For this review, take the finished solid that the model builds, in its own axes (mm). A direction names the side the tool comes from. Give positions to 0.01 mm unless a question says otherwise; leave off trailing zeros. Write each loop counter-clockwise with the first axis right and the second up, starting at its lowest first coordinate (ties: lowest second). Pieces come first, ordered by that corner, then holes. Notation, with made-up numbers: M 48.25,71 L 92.25,71 A19 cw 92.25,106 Z; hole C -22.5,38.5 d11. An arc over 180 degrees is marked long. Use one line per item in the form item = value. Start each with the question number.
Q1. Tool access review of faces 4 (the flat face through (-105.481, 72, 13)), 5 (the flat face through (52.164, 72, 13)), 6 (the flat face through (-35, 34.681, 13)): name each direction out of +Z, -Z, +X, -X, +Y, -Y from which nothing blocks a thin tool from reaching the whole face with its end or side.
Q2. Consider section A-A on x = -93.5. Write out the cut boundary in (y, z), and give its area (3 significant figures).
Q3. Consider section B-B on x = -15.5. Write out the cut boundary in (y, z).
Q4. Mouldability with a two-part tool opening along Y and no side actions: class faces 1 (the flat face through (-82.164, 41.556, 12.522)), 2 (the flat face through (57, 68.409, 13)), 3 (the flat face through (96.602, 51, 13)) as released by +Y, released by -Y, zero draft, split by the parting line, or undercut.
Q5. Consider section D-D on z = 14.5. Give the number of separate pieces and of enclosed holes in the cut face, and give its area (3 significant figures).
Q6. For probe 1 along Y at (x, z) = (-95, 9.75); probe 2 along Y at (x, z) = (-21, 10.75); probe 3 along X at (y, z) = (45, 2.75), list the stretches that pass through material, from the lowest coordinate up. Write a range as [from, to].
Q7. Clearance check with flat-ended pins moving along their axes: pin 1 Ø2.5 at (x, z) = (-22, 11) entering from -Y; pin 2 Ø8 at (y, z) = (72, 16) entering from -X; pin 3 Ø4 at (y, z) = (24.5, 18.5) entering from +X. State where each tip first meets the part, or that it passes through.
Q8. Consider section C-C on y = 65. Write out the cut boundary in (x, z).
```python
from build123d import *

# Parameters (mm, degrees)
F1_DEPTH = 7.62
F2_DEPTH = 25.4


with BuildPart() as f1:
    # F0 (on Top) → F1 (new body)
    with BuildSketch(Plane.XY):
        Polygon((-105.48081249, 68.0660605431), (-111.8125319481, 68.0660605431), (-111.8125319481, -59.1440834105), (-23.6834976822, -59.1440834105), (-23.6834976822, -53.6785013974), (-18.3922555298, -53.6785013974), (-18.3922555298, -59.1440834105), (57.8856468201, -59.1440834105), (57.8856468201, 26.6896747053), (96.6019257903, 26.6896747053), (96.6019257903, 75.7354423404), (61.1912831664, 75.7354423404), (61.1912831664, 68.4091001749), (52.1640814841, 68.4091001749), (52.1640814841, 75.83681494), (-105.48081249, 75.83681494), align=None)
        Polygon((-81.554395719, 53.1338888759), (-69.9187490924, 34.6805937588), (-77.8883700696, 34.6805937588), (-86.5607667147, 48.6274304688), (-89.5240166962, 46.4973681349), (-89.5240166962, 34.6805937588), (-96.544528266, 34.6805937588), (-96.544528266, 67.7835012539), (-89.5240166962, 67.7835012539), (-89.5240166962, 52.6339762873), (-86.7636297941, 56.5318454561), (-77.7941836398, 67.7835012539), (-70.0056904122, 67.7835012539), align=None, mode=Mode.SUBTRACT)
        with BuildLine():
            add(Edge.make_bspline(
                [(-49.8135689001, 34.6661035389), (-51.8711801342, 34.2241518301), (-54.8416752257, 34.2241518301)],
                knots=[0, 0, 0, 1, 1, 1], degree=2))
            add(Edge.make_bspline(
                [(-54.8416752257, 34.2241518301), (-60.9493029381, 34.2241518301), (-64.3907301783, 37.6003730804)],
                knots=[0, 0, 0, 1, 1, 1], degree=2))
            add(Edge.make_bspline(
                [(-64.3907301783, 37.6003730804), (-67.8321574184, 40.9765943308), (-67.8321574184, 47.156673143)],
                knots=[0, 0, 0, 1, 1, 1], degree=2))
            add(Edge.make_bspline(
                [(-67.8321574184, 47.156673143), (-67.8321574184, 53.5178797048), (-64.6515541375, 56.9919099398)],
                knots=[0, 0, 0, 1, 1, 1], degree=2))
            add(Edge.make_bspline(
                [(-64.6515541375, 56.9919099398), (-61.4709508566, 60.4659401749), (-55.8559906228, 60.4659401749)],
                knots=[0, 0, 0, 1, 1, 1], degree=2))
            add(Edge.make_bspline(
                [(-55.8559906228, 60.4659401749), (-50.4946092381, 60.4659401749), (-47.5060013717, 57.4121263186)],
                knots=[0, 0, 0, 1, 1, 1], degree=2))
            add(Edge.make_bspline(
                [(-47.5060013717, 57.4121263186), (-44.5173935053, 54.3583124624), (-44.5173935053, 48.9679506378)],
                knots=[0, 0, 0, 1, 1, 1], degree=2))
            Line((-44.5173935053, 48.9679506378), (-44.5173935053, 45.6134647175))
            Line((-44.5173935053, 45.6134647175), (-60.8406262885, 45.6134647175))
            add(Edge.make_bspline(
                [(-60.8406262885, 45.6134647175), (-60.7247045288, 42.6719500659), (-59.0945547835, 41.0200649906)],
                knots=[0, 0, 0, 1, 1, 1], degree=2))
            add(Edge.make_bspline(
                [(-59.0945547835, 41.0200649906), (-57.4644050381, 39.3681799154), (-54.5228903866, 39.3681799154)],
                knots=[0, 0, 0, 1, 1, 1], degree=2))
            add(Edge.make_bspline(
                [(-54.5228903866, 39.3681799154), (-52.2334356331, 39.3681799154), (-50.197559729, 39.842734619)],
                knots=[0, 0, 0, 1, 1, 1], degree=2))
            add(Edge.make_bspline(
                [(-50.197559729, 39.842734619), (-48.1616838248, 40.3172893227), (-45.9446801712, 41.3605851597)],
                knots=[0, 0, 0, 1, 1, 1], degree=2))
            Line((-45.9446801712, 41.3605851597), (-45.9446801712, 36.013693995))
            add(Edge.make_bspline(
                [(-45.9446801712, 36.013693995), (-47.755957666, 35.1080552476), (-49.8135689001, 34.6661035389)],
                knots=[0, 0, 0, 1, 1, 1], degree=2))
        make_face(mode=Mode.SUBTRACT)
        Polygon((-23.3689174759, 53.1338888759), (-11.7332708493, 34.6805937588), (-19.7028918265, 34.6805937588), (-28.3752884716, 48.6274304688), (-31.3385384531, 46.4973681349), (-31.3385384531, 34.6805937588), (-38.3590500229, 34.6805937588), (-38.3590500229, 67.7835012539), (-31.3385384531, 67.7835012539), (-31.3385384531, 52.6339762873), (-28.578151551, 56.5318454561), (-19.6087053967, 67.7835012539), (-11.8202121691, 67.7835012539), align=None, mode=Mode.SUBTRACT)
    extrude(amount=F1_DEPTH)

    # F0 (on Top) → F2 (join)
    with BuildSketch(Plane.XY):
        Polygon((-105.48081249, 68.0660605431), (-111.8125319481, 68.0660605431), (-111.8125319481, -59.1440834105), (-23.6834976822, -59.1440834105), (-23.6834976822, -53.6785013974), (-18.3922555298, -53.6785013974), (-18.3922555298, -59.1440834105), (57.8856468201, -59.1440834105), (57.8856468201, 26.6896747053), (96.6019257903, 26.6896747053), (96.6019257903, 75.7354423404), (61.1912831664, 75.7354423404), (61.1912831664, 68.4091001749), (52.1640814841, 68.4091001749), (52.1640814841, 75.83681494), (-105.48081249, 75.83681494), align=None)
        Polygon((-81.554395719, 53.1338888759), (-69.9187490924, 34.6805937588), (-77.8883700696, 34.6805937588), (-86.5607667147, 48.6274304688), (-89.5240166962, 46.4973681349), (-89.5240166962, 34.6805937588), (-96.544528266, 34.6805937588), (-96.544528266, 67.7835012539), (-89.5240166962, 67.7835012539), (-89.5240166962, 52.6339762873), (-86.7636297941, 56.5318454561), (-77.7941836398, 67.7835012539), (-70.0056904122, 67.7835012539), align=None, mode=Mode.SUBTRACT)
        with BuildLine():
            add(Edge.make_bspline(
                [(-49.8135689001, 34.6661035389), (-51.8711801342, 34.2241518301), (-54.8416752257, 34.2241518301)],
                knots=[0, 0, 0, 1, 1, 1], degree=2))
            add(Edge.make_bspline(
                [(-54.8416752257, 34.2241518301), (-60.9493029381, 34.2241518301), (-64.3907301783, 37.6003730804)],
                knots=[0, 0, 0, 1, 1, 1], degree=2))
            add(Edge.make_bspline(
                [(-64.3907301783, 37.6003730804), (-67.8321574184, 40.9765943308), (-67.8321574184, 47.156673143)],
                knots=[0, 0, 0, 1, 1, 1], degree=2))
            add(Edge.make_bspline(
                [(-67.8321574184, 47.156673143), (-67.8321574184, 53.5178797048), (-64.6515541375, 56.9919099398)],
                knots=[0, 0, 0, 1, 1, 1], degree=2))
            add(Edge.make_bspline(
                [(-64.6515541375, 56.9919099398), (-61.4709508566, 60.4659401749), (-55.8559906228, 60.4659401749)],
                knots=[0, 0, 0, 1, 1, 1], degree=2))
            add(Edge.make_bspline(
                [(-55.8559906228, 60.4659401749), (-50.4946092381, 60.4659401749), (-47.5060013717, 57.4121263186)],
                knots=[0, 0, 0, 1, 1, 1], degree=2))
            add(Edge.make_bspline(
                [(-47.5060013717, 57.4121263186), (-44.5173935053, 54.3583124624), (-44.5173935053, 48.9679506378)],
                knots=[0, 0, 0, 1, 1, 1], degree=2))
            Line((-44.5173935053, 48.9679506378), (-44.5173935053, 45.6134647175))
            Line((-44.5173935053, 45.6134647175), (-60.8406262885, 45.6134647175))
            add(Edge.make_bspline(
                [(-60.8406262885, 45.6134647175), (-60.7247045288, 42.6719500659), (-59.0945547835, 41.0200649906)],
                knots=[0, 0, 0, 1, 1, 1], degree=2))
            add(Edge.make_bspline(
                [(-59.0945547835, 41.0200649906), (-57.4644050381, 39.3681799154), (-54.5228903866, 39.3681799154)],
                knots=[0, 0, 0, 1, 1, 1], degree=2))
            add(Edge.make_bspline(
                [(-54.5228903866, 39.3681799154), (-52.2334356331, 39.3681799154), (-50.197559729, 39.842734619)],
                knots=[0, 0, 0, 1, 1, 1], degree=2))
            add(Edge.make_bspline(
                [(-50.197559729, 39.842734619), (-48.1616838248, 40.3172893227), (-45.9446801712, 41.3605851597)],
                knots=[0, 0, 0, 1, 1, 1], degree=2))
            Line((-45.9446801712, 41.3605851597), (-45.9446801712, 36.013693995))
            add(Edge.make_bspline(
                [(-45.9446801712, 36.013693995), (-47.755957666, 35.1080552476), (-49.8135689001, 34.6661035389)],
                knots=[0, 0, 0, 1, 1, 1], degree=2))
        make_face(mode=Mode.SUBTRACT)
        Polygon((-23.3689174759, 53.1338888759), (-11.7332708493, 34.6805937588), (-19.7028918265, 34.6805937588), (-28.3752884716, 48.6274304688), (-31.3385384531, 46.4973681349), (-31.3385384531, 34.6805937588), (-38.3590500229, 34.6805937588), (-38.3590500229, 67.7835012539), (-31.3385384531, 67.7835012539), (-31.3385384531, 52.6339762873), (-28.578151551, 56.5318454561), (-19.6087053967, 67.7835012539), (-11.8202121691, 67.7835012539), align=None, mode=Mode.SUBTRACT)
    extrude(amount=F2_DEPTH)


solid = f1.part
```
Working result:
q1.face_4 = +Z, -Z, -X, +Y
q1.face_5 = +Z, -Z, +Y
q1.face_6 = +Z, -Z
q2.outline = M -59.14,0 L 34.68,0 L 34.68,25.4 L -59.14,25.4 Z; M 67.78,0 L 75.84,0 L 75.84,25.4 L 67.78,25.4 Z
q2.area = 2,590 mm²
q3.outline = M -59.14,0 L 34.68,0 L 34.68,25.4 L -59.14,25.4 Z; M 40.65,0 L 63.12,0 L 63.12,25.4 L 40.65,25.4 Z; M 67.78,0 L 75.84,0 L 75.84,25.4 L 67.78,25.4 Z
q4.face_1 = undercut
q4.face_2 = released by +Y
q4.face_3 = zero draft
q5.separate_pieces = 1
q5.enclosed_holes = 3
q5.area = 23,200 mm²
q6.probe_1 = [-59.14, 34.68], [67.78, 75.84]
q6.probe_2 = [-53.68, 36.77], [49.38, 56.14], [66.04, 75.84]
q6.probe_3 = [-111.81, -96.54], [-89.52, -84.31], [-76.43, -67.72], [-60.8, -38.36], [-31.34, -26.12], [-18.24, 96.6]
q7.pin_1 = -53.68
q7.pin_2 = -111.81
q7.pin_3 = 57.89
q8.outline = M -111.81,0 L -96.54,0 L -96.54,25.4 L -111.81,25.4 Z; M -89.52,0 L -80.01,0 L -80.01,25.4 L -89.52,25.4 Z; M -72.2,0 L -38.36,0 L -38.36,25.4 L -72.2,25.4 Z; M -31.34,0 L -21.83,0 L -21.83,25.4 L -31.34,25.4 Z; M -14.01,0 L 96.6,0 L 96.6,25.4 L -14.01,25.4 Z
